Can you work these out from the model? Positions are in its coordinate system, mm. A direction names the side the tool comes from. Give positions to 0.01 mm unless a question says otherwise; leave off trailing zeros. Loops run counter-clockwise (first coordinate to the right, second up) from the corner with the lowest first, then second, coordinate; pieces in that order, holes last. Notation, with made-up numbers: M -10.5,21.5 L -1.5,21.5 A29 cw -1.5,50.5 Z; hole C 10,-26.5 d5. An arc over 180 degrees is marked long. Use CSV: the item, a comma, the result in double quotes.
from build123d import *

# Parameters (mm, degrees)
BOSS_EXTRUDE1_DEPTH        = 25.4
SKETCH2_W                  = 25.4
SKETCH2_H                  = 12.7
BOSS_EXTRUDE2_DEPTH        = 38.1
SKETCH3_W                  = 25.4
SKETCH3_H                  = 12.7
BOSS_EXTRUDE3_DEPTH        = 38.1
F_0_328IN_DOWEL_HOLE1_D    = 8.3312
F_0_55IN_DOWEL_HOLE2_D     = 13.8938
F_0_55IN_DOWEL_HOLE2_DEPTH = 35.052
F_0_55IN_DOWEL_HOLE2_TIP   = 4.174118634
FILLET1_R                  = 3.175
SKETCH8_W                  = 25.4
SKETCH8_H                  = 25.4
BOSS_EXTRUDE4_DEPTH        = 12.7
BOSS_EXTRUDE5_DEPTH        = 38.1
SKETCH9_W                  = 25.4
SKETCH9_H                  = 25.4
BOSS_EXTRUDE6_DEPTH        = 12.7
BOSS_EXTRUDE7_DEPTH        = 38.1


with BuildPart() as part:
    # Sketch1 → Boss-Extrude1 (new body)
    with BuildSketch(Plane.XY):
        Polygon((0, 0), (0, 53.34), (-61.591726717, 53.34), (0, 88.9), (25.4, 88.9), (86.991726717, 53.34), (25.4, 53.34), (25.4, 0), align=None)
    extrude(amount=BOSS_EXTRUDE1_DEPTH)

    # Sketch2 → Boss-Extrude2 (add)
    with BuildSketch(Plane.XY.offset(25.4)):
        with Locations((12.7, 6.35)):
            Rectangle(SKETCH2_W, SKETCH2_H)
    extrude(amount=BOSS_EXTRUDE2_DEPTH)

    # Sketch3 → Boss-Extrude3 (add)
    with BuildSketch(Plane(origin=(0, 0, 0), x_dir=(-1, 0, 0), z_dir=(0, 0, -1))):
        with Locations((-12.7, 6.35)):
            Rectangle(SKETCH3_W, SKETCH3_H)
    extrude(amount=BOSS_EXTRUDE3_DEPTH)

    # Ø0.328in Dowel Hole1 (through all)
    with Locations(Plane(origin=(0, 12.7, 0), x_dir=(1, 0, 0), z_dir=(0, 1, 0))):
        with Locations((12.7, 25.4), (12.7, -50.8)):
            Hole(F_0_328IN_DOWEL_HOLE1_D / 2)

    # Ø0.55in Dowel Hole2
    with Locations(Plane(origin=(0, 88.9, 0), x_dir=(1, 0, 0), z_dir=(0, 1, 0))):
        with Locations((12.7, -12.7)):
            Hole(F_0_55IN_DOWEL_HOLE2_D / 2, depth=F_0_55IN_DOWEL_HOLE2_DEPTH)
            with Locations((0, 0, -(F_0_55IN_DOWEL_HOLE2_DEPTH + F_0_55IN_DOWEL_HOLE2_TIP / 2))):  # 118° drill point
                Cone(0, F_0_55IN_DOWEL_HOLE2_D / 2, F_0_55IN_DOWEL_HOLE2_TIP, mode=Mode.SUBTRACT)

    # Fillet1
    fillet1_edges = [part.edges().sort_by_distance(p)[0] for p in [
        (0, 53.34, 12.7),
        (25.4, 53.34, 12.7),
    ]]
    fillet(fillet1_edges, radius=FILLET1_R)

    # Sketch8 → Boss-Extrude4 (add)
    with BuildSketch(Plane.XY.offset(25.4)):
        with Locations((12.7, 25.4)):
            Rectangle(SKETCH8_W, SKETCH8_H)
    extrude(amount=BOSS_EXTRUDE4_DEPTH)

    # Sketch8<3> → Boss-Extrude5 (add)
    with BuildSketch(Plane.XY.offset(25.4)):
        Polygon((0, 50.165), (0, 38.1), (25.4, 38.1), (25.4, 76.2), (0, 76.2), align=None)
    extrude(amount=BOSS_EXTRUDE5_DEPTH)

    # Sketch9 → Boss-Extrude6 (add)
    with BuildSketch(Plane(origin=(0, 0, 0), x_dir=(-1, 0, 0), z_dir=(0, 0, -1))):
        with Locations((-12.7, 25.4)):
            Rectangle(SKETCH9_W, SKETCH9_H)
    extrude(amount=BOSS_EXTRUDE6_DEPTH)

    # Sketch9<3> → Boss-Extrude7 (add)
    with BuildSketch(Plane(origin=(0, 0, 0), x_dir=(-1, 0, 0), z_dir=(0, 0, -1))):
        Polygon((-25.4, 50.165), (-25.4, 38.1), (0, 38.1), (0, 50.165), (0, 76.2), (-25.4, 76.2), align=None)
    extrude(amount=BOSS_EXTRUDE7_DEPTH)


solid = part.part
Q1. I want a section at A-A, the plane z = -25.4. Please give me the cut outline in (x, y), then the cut area to 3 significant figures.
Model answer:
outline,"M 0,0 L 8.53,0 L 8.53,12.7 L 0,12.7 Z; M 0,38.1 L 25.4,38.1 L 25.4,76.2 L 0,76.2 Z; M 16.87,0 L 25.4,0 L 25.4,12.7 L 16.87,12.7 Z"
area,"1,180 mm2"
Q2. I want a section at B-B, the plane y = 80. Please give me the cut outline in (x, z).
Model answer:
outline,"M -15.42,0 L 40.82,0 L 40.82,25.4 L -15.42,25.4 Z; hole C 12.7,12.7 d13.89"
Q3. For faces 1 (the flat face through (16, 12.7, -22)), 2 (the cylindrical face through (9.49, 71.13, 18.86)), 3 (the flat face through (13, 76.2, -19)), 4 (the flat face through (13, 76.2, 44)), which set-ups out of +Z, -Z, +X, -X, +Y, -Y let a thin tool reach every point of the face, with its end or its side?
Model answer:
face 1,"-Z, +X, -X"
face 2,"+Y"
face 3,"-Z, +X, -X, +Y"
face 4,"+Z, +X, -X, +Y"
Q4. If we mould it in two halves opening along Y, with no side actions, what happens to faces 5 (the flat face through (18, 88.9, 7)), 6 (the flat face through (13, 12.7, 45)), 7 (the flat face through (0, 38, 13))? For each: released by +Y, released by -Y, zero draft, split by the parting line, or undercut.
Model answer:
face 5,"released by +Y"
face 6,"undercut"
face 7,"zero draft"
Q5. I want a section at C-C, the plane x = 74. Please give me the cut outline in (y, z).
Model answer:
outline,"M 53.34,0 L 60.84,0 L 60.84,25.4 L 53.34,25.4 Z"
Q6. I'm going to push flat-ended pins straight in: P1, Ø1, axis at y = 31, z = 10.5, coming from the -X side; P2, Ø4, axis at x = -29, z = 6, coming from the +Y side; P3, Ø20.5, axis at x = 63, z = 18.5, coming from the -Y side. Where does each tip first touch, or does it pass through?
Model answer:
P1,"x = 0"
P2,"y = 73.31"
P3,"y = 53.34"
Q7. I want a section at D-D, the plane y = 45. Please give me the cut outline in (x, z).
Model answer:
outline,"M 0,-38.1 L 25.4,-38.1 L 25.4,63.5 L 0,63.5 Z"
Q8. Please list where these lines run through material, in increasing order: L1, parallel to Z at x = 12.7, y = 9; L2, parallel to Z at x = 12, y = 3; L3, parallel to X at y = 6.75, z = 50.8. Write a range as from..to.
Model answer:
L1,"-38.1..-29.57, -21.23..46.63, 54.97..63.5"
L2,"-38.1..-29.51, -21.29..46.69, 54.91..63.5"
L3,"0..8.53, 16.87..25.4"
